```python
from build123d import *

# Parameters (mm, degrees)
BOSS_EXTRUDE1_DEPTH                                 = 221.5
CSK_FOR_M3_COUNTERSUNK_FLAT_HEAD_SCREW1_D           = 3
CSK_FOR_M3_COUNTERSUNK_FLAT_HEAD_SCREW1_CSINK_D     = 5.5
CSK_FOR_M3_COUNTERSUNK_FLAT_HEAD_SCREW1_CSINK_ANGLE = 90
CSK_FOR_M3_COUNTERSUNK_FLAT_HEAD_SCREW4_D           = 3
CSK_FOR_M3_COUNTERSUNK_FLAT_HEAD_SCREW4_CSINK_D     = 5.5
CSK_FOR_M3_COUNTERSUNK_FLAT_HEAD_SCREW4_CSINK_ANGLE = 90
SKETCH12_W                                          = 8
SKETCH12_H                                          = 7
BOSS_EXTRUDE2_DEPTH                                 = 5.5
CUT_EXTRUDE1_DEPTH                                  = 359
BOSS_EXTRUDE3_DEPTH                                 = 3
BOSS_EXTRUDE4_DEPTH                                 = 2.5
BOSS_EXTRUDE4_DEPTH_BACK                            = 6
SKETCH19_W                                          = 0.6
SKETCH19_H                                          = 227
CUT_EXTRUDE2_DEPTH                                  = 10
SKETCH20_W                                          = 15.604741464
SKETCH20_H                                          = 2
CUT_EXTRUDE3_DEPTH                                  = 10
SKETCH21_W                                          = 0.6
SKETCH21_H                                          = 225
CUT_EXTRUDE4_DEPTH                                  = 10
SKETCH22_W                                          = 8.4
SKETCH22_H                                          = 5.5
CUT_EXTRUDE5_DEPTH                                  = 10
BOSS_EXTRUDE5_DEPTH                                 = 2
BOSS_EXTRUDE6_DEPTH                                 = 221.5
FILLET1_R                                           = 1


with BuildPart() as part:
    # Sketch1 → Boss-Extrude1 (new body)
    with BuildSketch(Plane(origin=(0, 0, 0), x_dir=(1, 0, 0), z_dir=(0, 1, 0))):
        Polygon((0, 0), (0, 9), (9, 9), (9, 7), (2, 7), (2, 0), align=None)
    extrude(amount=BOSS_EXTRUDE1_DEPTH)

    # CSK for M3 Countersunk Flat Head Screw1 (through all)
    with Locations(Plane.ZY):
        with Locations((-4, 211), (-4, 40.25)):
            CounterSinkHole(CSK_FOR_M3_COUNTERSUNK_FLAT_HEAD_SCREW1_D / 2, CSK_FOR_M3_COUNTERSUNK_FLAT_HEAD_SCREW1_CSINK_D / 2, counter_sink_angle=CSK_FOR_M3_COUNTERSUNK_FLAT_HEAD_SCREW1_CSINK_ANGLE)

    # CSK for M3 Countersunk Flat Head Screw4 (through all)
    with Locations(Plane(origin=(0, 0, -9), x_dir=(-1, 0, 0), z_dir=(0, 0, -1))):
        with Locations((-5, 10.25), (-5, 120)):
            CounterSinkHole(CSK_FOR_M3_COUNTERSUNK_FLAT_HEAD_SCREW4_D / 2, CSK_FOR_M3_COUNTERSUNK_FLAT_HEAD_SCREW4_CSINK_D / 2, counter_sink_angle=CSK_FOR_M3_COUNTERSUNK_FLAT_HEAD_SCREW4_CSINK_ANGLE)

    # Sketch12 → Boss-Extrude2 (add)
    with BuildSketch(Plane.XZ):
        with Locations((5, -3.5)):
            Rectangle(SKETCH12_W, SKETCH12_H)
    extrude(amount=-BOSS_EXTRUDE2_DEPTH)

    # Sketch13 → Cut-Extrude1 (cut)
    with BuildSketch(Plane(origin=(0, 221.5, 0), x_dir=(1, 0, 0), z_dir=(0, 1, 0))):
        Polygon((0, 8), (1, 9), (0, 9), align=None)
    extrude(amount=-CUT_EXTRUDE1_DEPTH, mode=Mode.SUBTRACT)

    # Sketch14 → Boss-Extrude3 (add)
    with BuildSketch(Plane.XZ):
        Polygon((0, 0), (9, 0), (9, -9), (1, -9), (0, -8), align=None)
    extrude(amount=BOSS_EXTRUDE3_DEPTH)

    # Sketch18 → Boss-Extrude4 (add, two sides: drawn at the far end of the back side and taken through both)
    with BuildSketch(Plane(origin=(0, 221.5, 0), x_dir=(1, 0, 0), z_dir=(0, 1, 0)).offset(-BOSS_EXTRUDE4_DEPTH_BACK)):
        Polygon((0, 0), (9, 0), (9, 9), (1, 9), (0, 8), align=None)
    extrude(amount=BOSS_EXTRUDE4_DEPTH + BOSS_EXTRUDE4_DEPTH_BACK)

    # Sketch19 → Cut-Extrude2 (cut)
    with BuildSketch(Plane.ZY):
        with Locations((-0.3, 110.5)):
            Rectangle(SKETCH19_W, SKETCH19_H)
    extrude(amount=-CUT_EXTRUDE2_DEPTH, mode=Mode.SUBTRACT)

    # Sketch20 → Cut-Extrude3 (cut)
    with BuildSketch(Plane.ZY):
        with Locations((-8.402370732, 223)):
            Rectangle(SKETCH20_W, SKETCH20_H)
    extrude(amount=-CUT_EXTRUDE3_DEPTH, mode=Mode.SUBTRACT)

    # Sketch21 → Cut-Extrude4 (cut)
    with BuildSketch(Plane(origin=(0, 0, -9), x_dir=(-1, 0, 0), z_dir=(0, 0, -1))):
        with Locations((-8.7, 109.5)):
            Rectangle(SKETCH21_W, SKETCH21_H)
    extrude(amount=-CUT_EXTRUDE4_DEPTH, mode=Mode.SUBTRACT)

    # Sketch22 → Cut-Extrude5 (cut)
    with BuildSketch(Plane(origin=(0, 0, -9), x_dir=(-1, 0, 0), z_dir=(0, 0, -1))):
        with Locations((-4.2, -0.25)):
            Rectangle(SKETCH22_W, SKETCH22_H)
    extrude(amount=-CUT_EXTRUDE5_DEPTH, mode=Mode.SUBTRACT)

    # Sketch26 → Boss-Extrude5 (add)
    with BuildSketch(Plane.XZ.offset(-2.5)):
        Polygon((8.4, -9), (8.4, -0.6), (0, -0.6), (0, -8), (1, -9), align=None)
    extrude(amount=BOSS_EXTRUDE5_DEPTH)

    # Sketch29 → Boss-Extrude6 (add)
    with BuildSketch(Plane(origin=(0, 222, 0), x_dir=(1, 0, 0), z_dir=(0, 1, 0))):
        Polygon((0, 8), (1, 9), (0, 9), align=None)
    extrude(amount=-BOSS_EXTRUDE6_DEPTH)

    # Fillet1
    fillet1_edges = [part.edges().sort_by_distance(p)[0] for p in [
        (0, 111.25, -9),
    ]]
    fillet(fillet1_edges, radius=FILLET1_R)


solid = part.part
```
The listing builds one solid part. Answer for the finished solid, in the listing's coordinates (mm). A direction names the side the tool comes from. Round coordinates to 2 decimals unless told otherwise and drop trailing zeros. Write each loop counter-clockwise with the first axis right and the second up, starting at its lowest first coordinate (ties: lowest second). Pieces come first, ordered by that corner, then holes. Notation, with made-up numbers: (74.5, 22) -> (126.5, 22) arc R20 cw to (126.5, 35) -> close; hole circle Ø5 at (35, 48). An arc over 180 degrees is marked (long way). Use CSV: the item, a comma, the result in double quotes. Start each with the question number.
(1) Section A-A on z = -4 is taken. Give the vertices of the cut face in (x, y), then the cut area to 3 significant figures.
(2) Each of these flat-tipped pins is pushed along its axis until it touches: pin 1 (2.5 mm diameter, centred on y = 211, z = -4, fed in from -X); pin 2 (5 mm diameter, centred on y = 40.25, z = -4, fed in from -X); pin 3 (3 mm diameter, centred on y = 150, z = -4, fed in from +X); pin 4 (5 mm diameter, centred on x = 5, y = 10.25, fed in from -Z). Where does it stop, or does it pass through?
(3) Section B-B on y = 194 is taken. Give the vertices of the cut face in (x, z), then the cut area to 3 significant figures.
(4) Which of the six approach directions +Z, -Z, +X, -X, +Y, -Y give full straight-line access (tool end or side, diameter ignored) to faces 1 (the face through (5, 5.5, -4)), 2 (the face through (8.4, 111.8, -7.3))?
(5) Consider L1, parallel to Y at x = 5, z = -7.6; L2, parallel to Y at x = 1.8, z = -4; L3, parallel to Z at x = 1.4, y = 40.25. Determine where each line is inside the solid, lowest interval first. Write a range as from..to.
A:
1,outline,"(0, 0.5) -> (8.4, 0.5) -> (8.4, 5.5) -> (2, 5.5) -> (2, 38.75) -> (1.25, 38.75) -> (0, 37.5) -> close; (0, 43) -> (1.25, 41.75) -> (2, 41.75) -> (2, 209.5) -> (1.25, 209.5) -> (0, 208.25) -> close; (0, 213.75) -> (1.25, 212.5) -> (2, 212.5) -> (2, 215.5) -> (8.4, 215.5) -> (8.4, 222) -> (0, 222) -> close"
1,area,"501 mm²"
2,pin 1,"passes through"
2,pin 2,"stops at x = 0.25"
2,pin 3,"stops at x = 2"
2,pin 4,"stops at z = -8.75"
3,outline,"(0, -8) arc R1 ccw to (1, -9) -> (8.4, -9) -> (8.4, -7) -> (2, -7) -> (2, -0.6) -> (0, -0.6) -> close"
3,area,"29.4 mm²"
4,face 1,"+Z, +X"
4,face 2,"+Z, -Z, +X, +Y, -Y"
5,L1,"y = 0.5..8.75, 11.75..118.5, 121.5..222"
5,L2,"y = 0.5..38.75, 41.75..209.5, 212.5..222"
5,L3,"z = -9..-5.5, -2.5..-0.6"
